Design review of the part built by this model. Coordinates are the model's own, in mm. Face numbers are marked on the shaded views. A direction names the side the tool comes from. Coordinates: 2 decimals unless noted, no trailing zeros. Loops run counter-clockwise (first coordinate to the right, second up) from the corner with the lowest first, then second, coordinate; pieces in that order, holes last.
Q1. Add section A-A on y = -50.5. Give the boundary of the cut face in (x, z).
Q2. For P1, Ø8, axis at x = 33, y = -51, coming from the +Z side; P2, Ø5.5, axis at x = 37.5, z = -12, coming from the +Y side; P3, Ø3.5, axis at x = 29, z = -4.5, coming from the +Y side; P4, Ø1.1, axis at x = 37, z = 2.5, coming from the +Y side, all flat-tipped, find the tip position at first contact; note any pin that passes through.
Q3. Add section D-D on y = -31.5. Give the boundary of the cut face in (x, z).
Q4. Add section C-C on z = -10. Give the boundary of the cut face in (x, y), and give its area (3 significant figures).
Q5. Machinability: for the marked faces 5, 6, 7 and 8, which of the approach directions +Z, -Z, +X, -X, +Y, -Y give a long, thin tool a straight path to every point of the face, cutting with its end or side? Answer none if there is none.
Q6. Wall thickness on probe 1 along Z at (x, y) = (34.5, -46); probe 2 along Y at (x, z) = (36.25, -7.25); probe 3 along Z at (x, y) = (41.25, -35.5): over which ranges is each line inside the solid? List them lowest first.
Q7. Add section B-B on z = 3.25. Give the boundary of the cut face in (x, y), and give its area (3 significant figures).
Q8. Draft analysis for pull direction X (two halves, no side actions). For the marked faces 1, 2, 3 and 4, state which applies: released by +X, released by -X, zero draft, split by the parting line, or undercut.
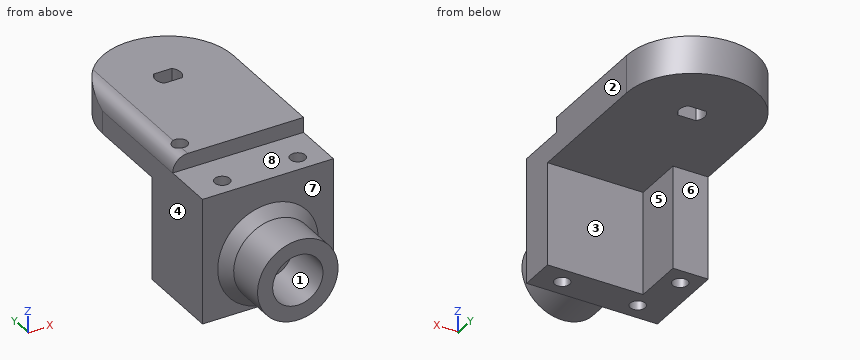
```python
from build123d import *

# Parameters (mm, degrees)
SKETCH1_W           = 26
SKETCH1_H           = 50
BOSS_EXTRUDE1_DEPTH = 8
SKETCH2_W           = 26
SKETCH2_H           = 50
BOSS_EXTRUDE2_DEPTH = 8
SKETCH3_W           = 26
SKETCH3_H           = 7
BOSS_EXTRUDE3_DEPTH = 36
SKETCH4_R           = 8
SKETCH4_R_2         = 5
BOSS_EXTRUDE4_DEPTH = 10
FILLET2_R           = 3
SKETCH6_W           = 7
SKETCH6_H           = 17
BOSS_EXTRUDE5_DEPTH = 20
CHAMFER1_SIZE       = 2
CUT_EXTRUDE2_DEPTH  = 0.5
CUT_EXTRUDE3_DEPTH  = 0.5
CUT_EXTRUDE4_START  = -36
CUT_EXTRUDE4_DEPTH  = 36
SKETCH11_W          = 26
SKETCH11_H          = 10
CUT_EXTRUDE5_DEPTH  = 3
SKETCH12_W          = 26
SKETCH12_H          = 10
CUT_EXTRUDE6_DEPTH  = 3
CUT_EXTRUDE7_REACH  = 90.986
SKETCH13_R          = 1.5
SKETCH14_W          = 39.670907723
SKETCH14_H          = 70.738486061
CUT_EXTRUDE8_DEPTH  = 8


with BuildPart() as part:
    # Sketch1 → Boss-Extrude1 (new body)
    with BuildSketch(Plane.XY):
        with Locations((37.264100782, -29)):
            Rectangle(SKETCH1_W, SKETCH1_H)
        with BuildLine():
            Line((39.049457889, -22.265997948), (35.478743675, -22.265997948))
            ThreePointArc((35.478743675, -22.265997948), (34.764100782, -20.515997948), (35.478743675, -18.765997947))
            Line((35.478743675, -18.765997947), (39.049457889, -18.765997947))
            ThreePointArc((39.049457889, -18.765997947), (39.764100782, -20.515997948), (39.049457889, -22.265997948))
        make_face(mode=Mode.SUBTRACT)
    extrude(amount=BOSS_EXTRUDE1_DEPTH)



with BuildPart() as body_2:
    # Sketch2 → Boss-Extrude2 (new body)
    with BuildSketch(Plane(origin=(0, 0, -20), x_dir=(-1, 0, 0), z_dir=(0, 0, -1))):
        with Locations((-37.264100782, -29)):
            Rectangle(SKETCH2_W, SKETCH2_H)
        with BuildLine():
            Line((-39.049457889, -18.765997947), (-35.478743675, -18.765997947))
            ThreePointArc((-35.478743675, -18.765997947), (-34.764100782, -20.515997948), (-35.478743675, -22.265997948))
            Line((-35.478743675, -22.265997948), (-39.049457889, -22.265997948))
            ThreePointArc((-39.049457889, -22.265997948), (-39.764100782, -20.515997948), (-39.049457889, -18.765997947))
        make_face(mode=Mode.SUBTRACT)
    extrude(amount=BOSS_EXTRUDE2_DEPTH)


with BuildPart() as part_1:
    add(part.part)

    add(body_2.part)  # Boss-Extrude3 merges body 2
    # Sketch3 → Boss-Extrude3 (add)
    with BuildSketch(Plane.XY.offset(8)):
        with Locations((37.264100782, -50.5)):
            Rectangle(SKETCH3_W, SKETCH3_H)
    extrude(amount=-BOSS_EXTRUDE3_DEPTH)

    # Sketch4 → Boss-Extrude4 (add)
    with BuildSketch(Plane.XZ.offset(54)):
        with Locations(Location((37.264100782, -10, 0), (0, 0, 90))):
            Circle(SKETCH4_R)
        with Locations(Location((37.264100782, -10, 0), (0, 0, 270))):
            Circle(SKETCH4_R_2, mode=Mode.SUBTRACT)
    extrude(amount=BOSS_EXTRUDE4_DEPTH)

    # Fillet2
    fillet2_edges = [part_1.edges().sort_by_distance(p)[0] for p in [
        (24.264100782, -29, 8),
        (24.264100782, -29, -28),
    ]]
    fillet(fillet2_edges, radius=FILLET2_R)

    # Sketch6 → Boss-Extrude5 (add)
    with BuildSketch(Plane.XY.offset(-20)):
        with Locations((27.764100782, -45.5)):
            Rectangle(SKETCH6_W, SKETCH6_H)
    extrude(amount=BOSS_EXTRUDE5_DEPTH)

    # Chamfer1
    chamfer1_edges = [part_1.edges().sort_by_distance(p)[0] for p in [
        (37.264100782, -54, -18),
    ]]
    chamfer(chamfer1_edges, length=CHAMFER1_SIZE)

    # Sketch7 → Cut-Extrude2 (cut)
    with BuildSketch(Plane(origin=(0, 0, 0), x_dir=(-1, 0, 0), z_dir=(0, 0, -1))):
        Polygon((-50.264100782, -4), (-50.264100782, -47), (-31.264100782, -47), (-31.264100782, -37), (-24.264100782, -37), (-24.264100782, -4), align=None)
    extrude(amount=-CUT_EXTRUDE2_DEPTH, mode=Mode.SUBTRACT)

    # Sketch8 → Cut-Extrude3 (cut)
    with BuildSketch(Plane.XY.offset(-20)):
        Polygon((50.264100782, -47), (50.264100782, -4), (24.264100782, -4), (24.264100782, -37), (31.264100782, -37), (31.264100782, -47), align=None)
    extrude(amount=-CUT_EXTRUDE3_DEPTH, mode=Mode.SUBTRACT)

    # Sketch10 → Cut-Extrude4 (cut)
    with BuildSketch(Plane.XY.offset(8).offset(CUT_EXTRUDE4_START)):
        with BuildLine():
            Line((50.264100782, -20.515997948), (50.264100782, 2.26582648))
            Line((50.264100782, 2.26582648), (24.264100782, 2.26582648))
            Line((24.264100782, 2.26582648), (24.264100782, -20.515997948))
            ThreePointArc((24.264100782, -20.515997948), (37.264100782, -7.515997948), (50.264100782, -20.515997948))
        make_face()
    extrude(amount=CUT_EXTRUDE4_DEPTH, mode=Mode.SUBTRACT)

    # Sketch11 → Cut-Extrude5 (cut)
    with BuildSketch(Plane.XY.offset(8)):
        with Locations((37.264100782, -49)):
            Rectangle(SKETCH11_W, SKETCH11_H)
    extrude(amount=-CUT_EXTRUDE5_DEPTH, mode=Mode.SUBTRACT)

    # Sketch12 → Cut-Extrude6 (cut)
    with BuildSketch(Plane(origin=(0, 0, -28), x_dir=(-1, 0, 0), z_dir=(0, 0, -1))):
        with Locations((-37.264100782, -49)):
            Rectangle(SKETCH12_W, SKETCH12_H)
    extrude(amount=-CUT_EXTRUDE6_DEPTH, mode=Mode.SUBTRACT)

    # Cut-Extrude7: up to this face of the body (flat: up to its plane)
    cut_extrude7_end = Plane(part_1.part.faces().sort_by_distance((38.560022368, -26.898937337, -28))[0])
    # Sketch13 → Cut-Extrude7 (cut, up to the picked face)
    with BuildSketch(Plane.XY.offset(8), mode=Mode.PRIVATE) as cut_extrude7_sk1:
        with Locations((45.264100782, -50.5)):
            Circle(SKETCH13_R)
    cut_extrude7_tool1 = split(extrude(cut_extrude7_sk1.sketch, amount=-CUT_EXTRUDE7_REACH, mode=Mode.PRIVATE), bisect_by=cut_extrude7_end, keep=Keep.BOTH, mode=Mode.PRIVATE)
    # Sketch13 → Cut-Extrude7 (cut, up to the picked face)
    with BuildSketch(Plane.XY.offset(8), mode=Mode.PRIVATE) as cut_extrude7_sk2:
        with Locations((30.264100782, -50.5)):
            Circle(SKETCH13_R)
    cut_extrude7_tool2 = split(extrude(cut_extrude7_sk2.sketch, amount=-CUT_EXTRUDE7_REACH, mode=Mode.PRIVATE), bisect_by=cut_extrude7_end, keep=Keep.BOTH, mode=Mode.PRIVATE)
    # Sketch13 → Cut-Extrude7 (cut, up to the picked face)
    with BuildSketch(Plane.XY.offset(8), mode=Mode.PRIVATE) as cut_extrude7_sk3:
        with Locations(Location((27.764100782, -40.5, 0), (0, 0, 109.471220634))):
            Circle(SKETCH13_R)
    cut_extrude7_tool3 = split(extrude(cut_extrude7_sk3.sketch, amount=-CUT_EXTRUDE7_REACH, mode=Mode.PRIVATE), bisect_by=cut_extrude7_end, keep=Keep.BOTH, mode=Mode.PRIVATE)
    add(cut_extrude7_tool1.solids().sort_by(Axis((45.264101, -50.5, 8), (0, 0, -1)))[0], mode=Mode.SUBTRACT)
    add(cut_extrude7_tool2.solids().sort_by(Axis((30.264101, -50.5, 8), (0, 0, -1)))[0], mode=Mode.SUBTRACT)
    add(cut_extrude7_tool3.solids().sort_by(Axis((27.764101, -40.5, 8), (0, 0, -1)))[0], mode=Mode.SUBTRACT)

    # Sketch14 → Cut-Extrude8 (cut)
    with BuildSketch(Plane(origin=(0, 0, -28), x_dir=(-1, 0, 0), z_dir=(0, 0, -1))):
        with Locations((-35.76618016, -37.229796089)):
            Rectangle(SKETCH14_W, SKETCH14_H)
    extrude(amount=-CUT_EXTRUDE8_DEPTH, mode=Mode.SUBTRACT)


solid = part_1.part
```
Entries:
1. outline: (24.26, -20) - (28.76, -20) - (28.76, 5) - (24.26, 5) - close; (31.76, -20) - (43.76, -20) - (43.76, 5) - (31.76, 5) - close; (46.76, -20) - (50.26, -20) - (50.26, 5) - (46.76, 5) - close
2. P1: stops at z = 5
2. P2: stops at y = -47
2. P3: stops at y = -37
2. P4: stops at y = -7.52
3. outline: (24.26, 0.5) - (50.26, 0.5) - (50.26, 8) - (27.26, 8) arc R3 ccw to (24.26, 5) - close
4. outline: (24.26, -54) - (27.26, -54) - (29.26, -56) - (29.26, -64) - (32.26, -64) - (32.26, -54) - (42.26, -54) - (42.26, -64) - (45.26, -64) - (45.26, -56) - (47.26, -54) - (50.26, -54) - (50.26, -47) - (31.26, -47) - (31.26, -37) - (24.26, -37) - close; hole circle Ø3 at (27.76, -40.5); hole circle Ø3 at (30.26, -50.5); hole circle Ø3 at (45.26, -50.5)
4. area: 295 mm2
5. face 5: -Z, +X, +Y
5. face 6: -Z, +X, -X, +Y
5. face 7: -Y
5. face 8: +Z, +X, -X, -Y
6. probe 1: z = 0.5 to 5
6. probe 2: y = -54 to -47
6. probe 3: z = 0.5 to 8
7. outline: (24.26, -54) - (50.26, -54) - (50.26, -20.52) arc R13 ccw to (24.26, -20.52) - close; hole circle Ø3 at (27.76, -40.5); hole circle Ø3 at (30.26, -50.5); hole (35.48, -22.27) - (39.05, -22.27) arc R2.5 ccw to (39.05, -18.77) - (35.48, -18.77) arc R2.5 ccw to start; hole circle Ø3 at (45.26, -50.5)
7. area: 1,100 mm2
8. face 1: undercut
8. face 2: released by +X
8. face 3: zero draft
8. face 4: released by -X
